from build123d import *

# Parameters (mm, degrees)
BOSS_EXTRUDE1_DEPTH = 250
SKETCH3_W           = 20
SKETCH3_H           = 20
CUT_EXTRUDE1_DEPTH  = 20


with BuildPart() as part:
    # Sketch1 → Boss-Extrude1 (new body)
    with BuildSketch(Plane.XY):
        Polygon((0, 15), (-15, 15), (-15, -15), (15, -15), (15, 15), align=None)
    extrude(amount=BOSS_EXTRUDE1_DEPTH)

    # Sketch3 → Cut-Extrude1 (cut)
    with BuildSketch(Plane(origin=(0, -15, 0), x_dir=(-1, 0, 0), z_dir=(0, -1, 0))):
        with Locations((0, -235)):
            Rectangle(SKETCH3_W, SKETCH3_H)
        with Locations((0, -15)):
            Rectangle(SKETCH3_W, SKETCH3_H)
    extrude(amount=-CUT_EXTRUDE1_DEPTH, mode=Mode.SUBTRACT)


solid = part.part
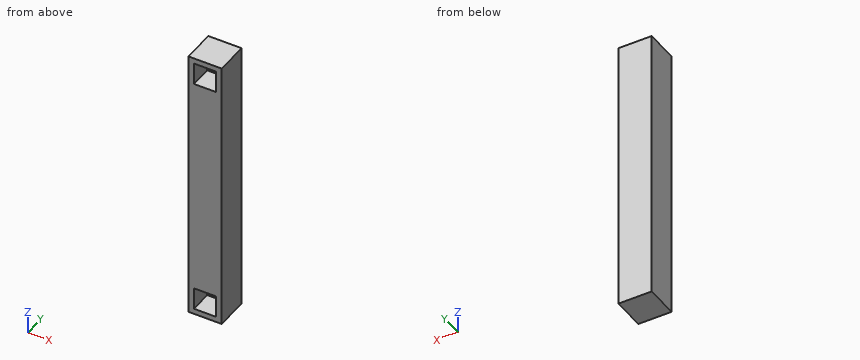
The model under review builds one solid part; all positions refer to its coordinate system, in mm. Give positions to 0.01 mm unless a question says otherwise; leave off trailing zeros. Order: outer loops, then holes, each group sorted by start corner. A loop starts at its lowest first (then second) coordinate and runs counter-clockwise, first axis right, second up. Notation, with made-up numbers: M -38,0 L -10,0 A24 cw -10,29 Z; hole C -31.75,36 d10. An arc over 180 degrees is marked long. Answer in a Markdown table with one row per item. Add a question column.
1. To check wall thickness, follow line 1 along Z through (x, y) = (6.5, 0.25); line 2 along X through (y, z) = (-6.5, 16); line 3 along Y through (x, z) = (-8, 234). State the ranges of each line that lie inside material, in increasing order.
2. Add section B-B on x = 6.25. State the section outline as (y, z) points, plus the area to 3 significant figures.
3. Add section A-A on y = -11.25. State the section outline as (x, z) points, plus the area to 3 significant figures.
4. For pin 1 Ø6 at (x, z) = (1, 15.5) entering from -Y, flat-tipped, find the tip position at first contact; note if it passes through.
The answers:
| question | item | result |
|---|---|---|
| 1 | line 1 | 0 to 5, 25 to 225, 245 to 250 |
| 1 | line 2 | -15 to -10, 10 to 15 |
| 1 | line 3 | 5 to 15 |
| 2 | outline | M -15,0 L 15,0 L 15,250 L -15,250 L -15,245 L 5,245 L 5,225 L -15,225 L -15,25 L 5,25 L 5,5 L -15,5 Z |
| 2 | area | 6,700 mm2 |
| 3 | outline | M -15,0 L 15,0 L 15,250 L -15,250 Z; hole M -10,5 L 10,5 L 10,25 L -10,25 Z; hole M -10,225 L 10,225 L 10,245 L -10,245 Z |
| 3 | area | 6,700 mm2 |
| 4 | pin 1 | y = 5 |
